Can you work these out from the model? Positions are in its coordinate system, mm. Face numbers are marked on the shaded views. A direction names the side the tool comes from. Coordinates: 2 decimals unless noted, no trailing zeros. Order: outer loops, then holes, each group sorted by start corner. A loop starts at its lowest first (then second) coordinate and runs counter-clockwise, first axis right, second up. Notation, with made-up numbers: (33, 44) - (91, 44) arc R29 ccw to (91, 77) - close; hole circle Ø7 at (-7, -31). An arc over 180 degrees is marked (long way). Use a Markdown table: item, result. Add a question column.
(1) On a 3-axis mill with a long thin cutter (end or side, diameter ignored), from which of +Z, -Z, +X, -X, +Y, -Y can I reach the whole of each face in a straight line? I mean the marked faces 5, 6 and 7. Say none if no direction works.
(2) We'd pull the mould along X, two halves only. Please class the marked faces 1, 2, 3 and 4: pulls with the +X half, pulls with the -X half, needs draft (parallel to the pull), parting line crosses it, or undercut.
(3) If I drill on L1, parallel to Y at x = -10, z = 3.5; L2, parallel to X at y = 43.5, z = 14.75; L3, parallel to Y at x = -32, z = 13.5, over which ranges is the centre line in solid material (lowest first)? Write a range as [from, to].
(4) I want a section at A-A (z = 16.5). List the corners of the cut face in (x, y) for me.
(5) I want a section at B-B (z = 2.25). State how many separate pieces and enclosed holes the cut face has, and give its area (3 significant figures).
(6) I want a section at C-C (y = 42). List the corners of the cut face in (x, z) for me, and give its area (3 significant figures).
(7) I want a section at D-D (x = -4.5). List the corners of the cut face in (y, z) for me, and give its area (3 significant figures).
(8) For pin 1 Ø2.5 at (x, y) = (-10, 25) entering from +Z; pin 2 Ø5.5 at (x, y) = (-10, 25) entering from -Z; pin 3 Ø6.5 at (x, y) = (-31.5, 23.5) entering from +Z, each with a flat end and sliding along its axis, tell me the tip position at first contact or that it passes through.
```python
from build123d import *

# Parameters (mm, degrees)
F0_W           = 40
F0_H           = 24
F1_DEPTH       = 8
F0_H_2         = 13
F2_DEPTH       = 20
F3_D           = 5
F5_DEPTH       = 5
F7_D           = 3
F7_CBORE_D     = 6
F7_CBORE_DEPTH = 1
F8_R           = 1.5
F9_DEPTH       = 3


with BuildPart() as f1:
    # F0 (on Top) → F1 (new body)
    with BuildSketch(Plane.XY):
        with Locations((-20, 25)):
            Rectangle(F0_W, F0_H)
    extrude(amount=F1_DEPTH)

    # F0 (on Top) → F2 (join)
    with BuildSketch(Plane.XY):
        with Locations((-20, 43.5)):
            Rectangle(F0_W, F0_H_2)
        with Locations((-20, 6.5)):
            Rectangle(F0_W, F0_H_2)
    extrude(amount=F2_DEPTH)

    # F3 (through all)
    with Locations(Plane(origin=(0, 0, 0), x_dir=(1, 0, 0), z_dir=(0, 0, -1))):
        with Locations((-8, -43.5), (-32, -43.5), (-32, -6.5), (-8, -6.5)):
            Hole(F3_D / 2)

    # F4 (on face) → F5 (cut)
    with BuildSketch(Plane.XY):
        Polygon((-29.6905989232, 10.5), (-34.3094010768, 10.5), (-36.6188021535, 6.5), (-34.3094010768, 2.5), (-29.6905989232, 2.5), (-27.3811978465, 6.5), align=None)
        Polygon((-5.6905989232, 10.5), (-10.3094010768, 10.5), (-12.6188021535, 6.5), (-10.3094010768, 2.5), (-5.6905989232, 2.5), (-3.3811978465, 6.5), align=None)
        Polygon((-5.6905989232, 47.5), (-10.3094010768, 47.5), (-12.6188021535, 43.5), (-10.3094010768, 39.5), (-5.6905989232, 39.5), (-3.3811978465, 43.5), align=None)
        Polygon((-29.6905989232, 47.5), (-34.3094010768, 47.5), (-36.6188021535, 43.5), (-34.3094010768, 39.5), (-29.6905989232, 39.5), (-27.3811978465, 43.5), align=None)
    extrude(amount=F5_DEPTH, mode=Mode.SUBTRACT)

    # F7 (through all)
    with Locations(Plane(origin=(0, 0, 0), x_dir=(1, 0, 0), z_dir=(0, 0, -1))):
        with Locations((-30, -25), (-10, -25)):
            CounterBoreHole(F7_D / 2, F7_CBORE_D / 2, F7_CBORE_DEPTH)

    # F8 (on face) → F9 (cut)
    with BuildSketch(Plane.XY.offset(8)):
        Polygon((-8.2679491924, 28), (-11.7320508076, 28), (-13.4641016151, 25), (-11.7320508076, 22), (-8.2679491924, 22), (-6.5358983849, 25), align=None)
        with Locations((-10, 25)):
            Circle(F8_R, mode=Mode.SUBTRACT)
        Polygon((-28.2679491924, 28), (-31.7320508076, 28), (-33.4641016151, 25), (-31.7320508076, 22), (-28.2679491924, 22), (-26.5358983849, 25), align=None)
        with Locations((-30, 25)):
            Circle(F8_R, mode=Mode.SUBTRACT)
    extrude(amount=-F9_DEPTH, mode=Mode.SUBTRACT)


solid = f1.part
```
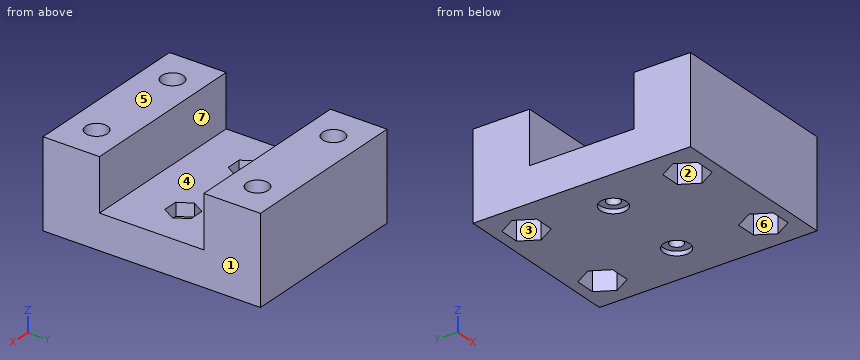
Answers follow:
| question | item | result |
|---|---|---|
| 1 | face 5 | +Z, +X, -X, +Y, -Y |
| 1 | face 6 | -Z |
| 1 | face 7 | +Z, +X, -X |
| 2 | face 1 | pulls with the +X half |
| 2 | face 2 | undercut |
| 2 | face 3 | undercut |
| 2 | face 4 | needs draft |
| 3 | L1 | y = [0, 2.5], [10.5, 23.5], [26.5, 39.5], [47.5, 50] |
| 3 | L2 | x = [-40, -34.5], [-29.5, -10.5], [-5.5, 0] |
| 3 | L3 | y = [0, 4], [9, 13], [37, 41], [46, 50] |
| 4 | outline | (-40, 0) - (0, 0) - (0, 13) - (-40, 13) - close; (-40, 37) - (0, 37) - (0, 50) - (-40, 50) - close; hole circle Ø5 at (-32, 6.5); hole circle Ø5 at (-32, 43.5); hole circle Ø5 at (-8, 6.5); hole circle Ø5 at (-8, 43.5) |
| 5 | separate pieces | 1 |
| 5 | enclosed holes | 6 |
| 5 | area | 1,760 mm² |
| 6 | outline | (-40, 0) - (-35.75, 0) - (-35.75, 5) - (-34, 5) - (-34, 20) - (-40, 20) - close; (-30, 5) - (-28.25, 5) - (-28.25, 0) - (-11.75, 0) - (-11.75, 5) - (-10, 5) - (-10, 20) - (-30, 20) - close; (-6, 5) - (-4.25, 5) - (-4.25, 0) - (0, 0) - (0, 20) - (-6, 20) - close |
| 6 | area | 605 mm² |
| 7 | outline | (0, 0) - (4.56, 0) - (4.56, 5) - (8.44, 5) - (8.44, 0) - (41.56, 0) - (41.56, 5) - (45.44, 5) - (45.44, 0) - (50, 0) - (50, 20) - (37, 20) - (37, 8) - (13, 8) - (13, 20) - (0, 20) - close |
| 7 | area | 673 mm² |
| 8 | pin 1 | passes through |
| 8 | pin 2 | stops at z = 1 |
| 8 | pin 3 | stops at z = 8 |
